Design review of the part shown in the three views and the two pictorial views. Dimensions are in mm from the part's minimum x, y and z. Round coordinates to 2 decimals unless told otherwise and drop trailing zeros. Loops run counter-clockwise (first coordinate to the right, second up) from the corner with the lowest first, then second, coordinate; pieces in that order, holes last. Notation, with made-up numbers: (-25.75, 49) -> (-6.75, 49) arc R11 ccw to (-6.75, 58) -> close; hole circle Ø3 at (-33, 75.5). An arc over 180 degrees is marked (long way). Use a Markdown table: item, result. Add a question column.
1) Insertion check: pin 1 (2 mm diameter, centred on x = 168, y = 22, fed in from -Z) (1 decimal); pin 2 (5.5 mm diameter, centred on x = 114.01, z = 62.07, fed in from +Y); pin 3 (4 mm diameter, centred on y = 2.5, z = 22, fed in from -X); pin 4 (4 mm diameter, centred on x = 105.5, y = 8.5, fed in from +Z). Each pin has a flat end and moves straight along its axis. Give the tip position at first contact, or say it passes through.
2) Consider section A-A on z = 95. Give the boundary of the cut face in (x, y) (1 decimal).
3) Wall thickness on probe 1 along X at (y, z) = (23.5, 95) (1 decimal); probe 2 along X at (y, z) = (7, 95); probe 3 along X at (y, z) = (12, 90): over which ranges is each line inside the solid? List them lowest first.
4) Consider section C-C on y = 22.75. Give the boundary of the cut face in (x, z).
5) Mouldability with a two-part tool opening along X and no side actions: class the marked faces 1, 2 and 3 as released by +X, released by -X, zero draft, split by the parting line, or undercut.
6) Consider section D-D on y = 3. Give the boundary of the cut face in (x, z).
7) Consider section B-B on x = 95. Give the boundary of the cut face in (y, z), plus the area to 4 significant figures.
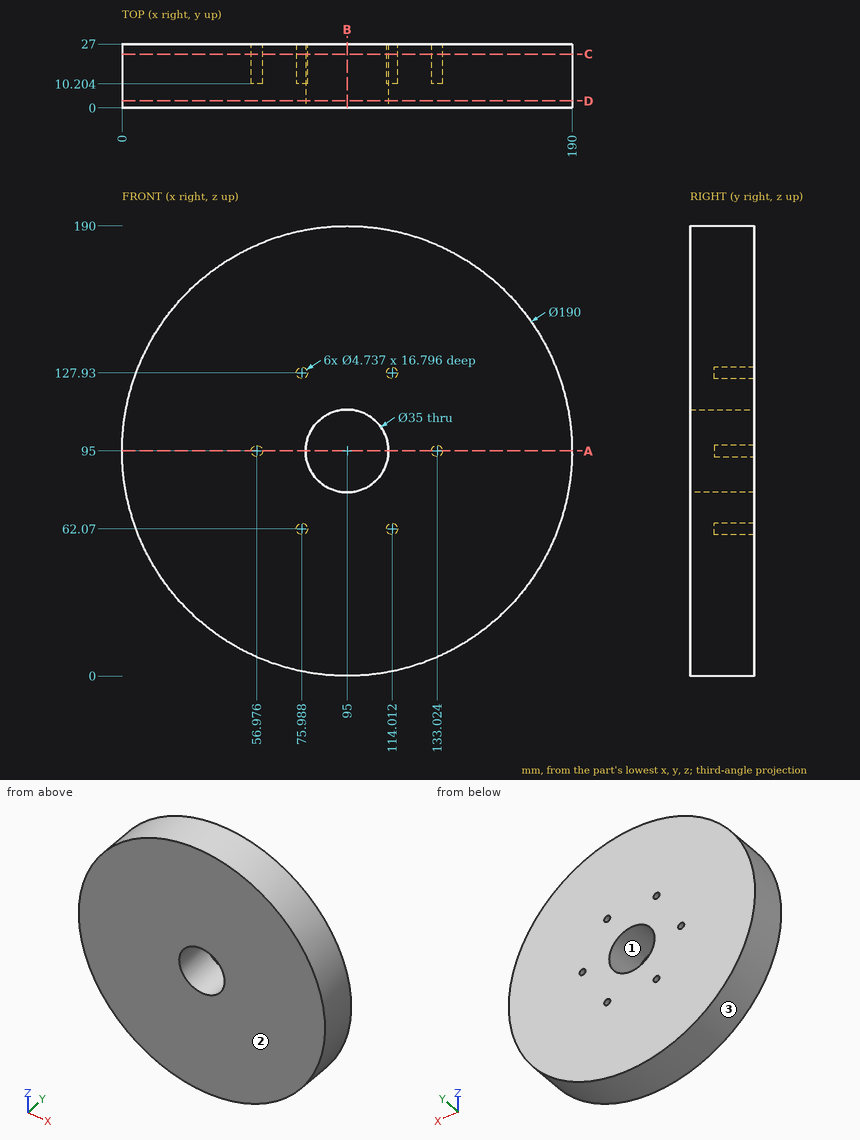
Result set:
| question | item | result |
|---|---|---|
| 1 | pin 1 | z = 33 |
| 1 | pin 2 | y = 27 |
| 1 | pin 3 | x = 31.88 |
| 1 | pin 4 | z = 189.62 |
| 2 | outline | (0, 0) -> (77.5, 0) -> (77.5, 27) -> (59.3, 27) -> (59.3, 10.2) -> (54.6, 10.2) -> (54.6, 27) -> (0, 27) -> close; (112.5, 0) -> (190, 0) -> (190, 27) -> (135.4, 27) -> (135.4, 10.2) -> (130.7, 10.2) -> (130.7, 27) -> (112.5, 27) -> close |
| 3 | probe 1 | 0 to 54.6, 59.3 to 77.5, 112.5 to 130.7, 135.4 to 190 |
| 3 | probe 2 | 0 to 77.5, 112.5 to 190 |
| 3 | probe 3 | 0.13 to 78.23, 111.77 to 189.87 |
| 4 | outline | circle Ø190 at (95, 95); hole circle Ø4.74 at (56.98, 95); hole circle Ø4.74 at (75.99, 62.07); hole circle Ø4.74 at (75.99, 127.93); hole circle Ø35 at (95, 95); hole circle Ø4.74 at (114.01, 62.07); hole circle Ø4.74 at (114.01, 127.93); hole circle Ø4.74 at (133.02, 95) |
| 5 | face 1 | undercut |
| 5 | face 2 | zero draft |
| 5 | face 3 | split by the parting line |
| 6 | outline | circle Ø190 at (95, 95); hole circle Ø35 at (95, 95) |
| 7 | outline | (0, 0) -> (27, 0) -> (27, 77.5) -> (0, 77.5) -> close; (0, 112.5) -> (27, 112.5) -> (27, 190) -> (0, 190) -> close |
| 7 | area | 4,185 mm2 |
